Verification items for this drawing (mm, ordinates from the low corner). A direction names the side the tool comes from. Give positions to 0.01 mm unless a question says otherwise; leave off trailing zeros. Loops run counter-clockwise (first coordinate to the right, second up) from the corner with the lowest first, then second, coordinate; pieces in that order, holes last. Notation, with made-up numbers: (2, 28.25) - (36, 28.25) arc R26 cw to (36, 67.25) - close; hole circle Ø5 at (30.25, 31). An arc over 180 degrees is marked (long way). Write item = value, one per line. Start each with the question number.
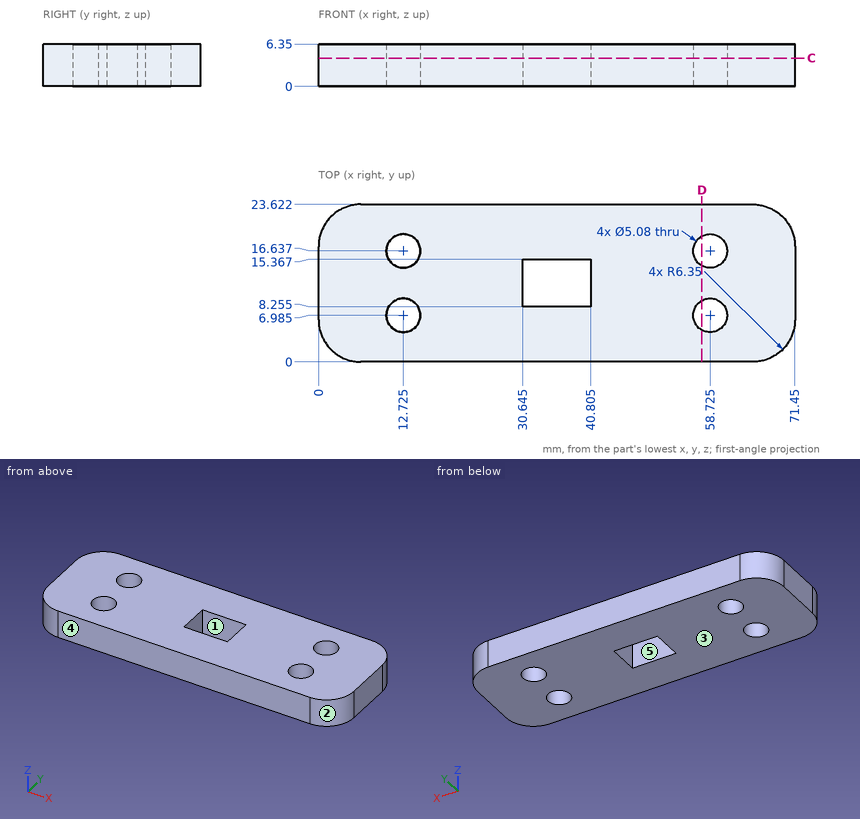
1) Material ranges on line 1 along X through (y, z) = (7.5, 2.5); line 2 along Y through (x, z) = (35, 5.5) (1 decimal); line 3 along X through (y, z) = (17.5, 0.5) (1 decimal), recorded low to high.
2) Gauge pin test, flat end, axial feed: P1, Ø2, axis at y = 20, z = 0.5, coming from the -X side. Record the tip position at first contact, or that the pin passes through.
3) Cross-section at D-D on x = 57.5. Enter the section's corners in (y, z).
4) Tool access check on the marked faces 1 and 2. Record the directions out of +Z, -Z, +X, -X, +Y, -Y that give a thin tool (end or side, any length) a straight path to the whole face; none if there is none.
5) Cross-section at C-C on z = 4.25. Give the number of separate pieces and of enclosed holes in the cut face, and give its area (3 significant figures).
6) Release check for a two-part mould opening along Y. For the marked faces 3, 4 and 5 record: pulls with the +Y half, pulls with the -Y half, needs draft (parallel to the pull), parting line crosses it, or undercut.
Checked values:
q1.line_1 = 0 to 10.24, 15.21 to 56.24, 61.21 to 71.45
q1.line_2 = 0 to 8.3, 15.4 to 23.6
q1.line_3 = 0 to 10.3, 15.1 to 56.3, 61.1 to 71.4
q2.P1 = 0.24
q3.outline = (0, 0) - (4.76, 0) - (4.76, 6.35) - (0, 6.35) - close; (9.21, 0) - (14.41, 0) - (14.41, 6.35) - (9.21, 6.35) - close; (18.86, 0) - (23.62, 0) - (23.62, 6.35) - (18.86, 6.35) - close
q4.face_1 = +Z, -Z
q4.face_2 = +Z, -Z, +X, -Y
q5.separate_pieces = 1
q5.enclosed_holes = 5
q5.area = 1,500 mm²
q6.face_3 = needs draft
q6.face_4 = pulls with the -Y half
q6.face_5 = undercut
